Check sheet for the modelled part. Datum: model origin and axes. Units: mm. Face numbers are marked on the shaded views. A direction names the side the tool comes from. Coordinates: 2 decimals unless noted, no trailing zeros. Loops run counter-clockwise (first coordinate to the right, second up) from the corner with the lowest first, then second, coordinate; pieces in that order, holes last. Notation, with made-up numbers: (47.25, -8) -> (89.25, -8) arc R17 ccw to (89.25, 12) -> close; hole circle Ø1 at (31.25, -23). An arc over 180 degrees is marked (long way). Use CSV: the item, a comma, the result in double quotes.
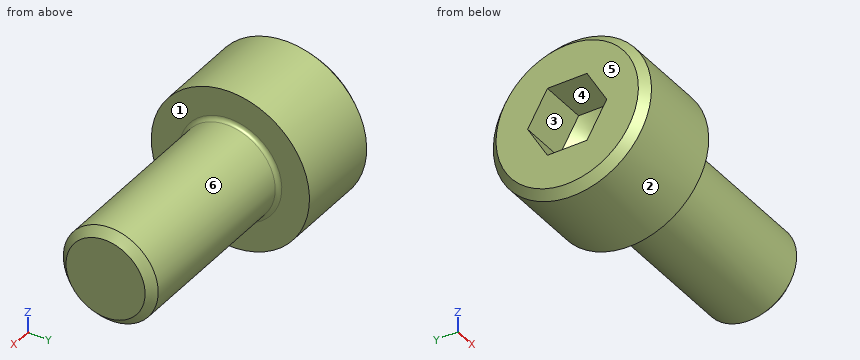
```python
from build123d import *

# Parameters (mm, degrees)
CHAMFER1_SIZE      = 0.5
CUT_EXTRUDE1_DEPTH = 3


with BuildPart() as part:
    # Sketch1 → Revolve1 (revolve)
    with BuildSketch(Plane.XY, mode=Mode.PRIVATE) as revolve1_sk:
        with BuildLine():
            Line((0, 0), (0, 5))
            Line((0, 5), (6, 5))
            Line((6, 5), (6, 3.25))
            ThreePointArc((6, 3.25), (6.073223305, 3.073223305), (6.25, 3))
            Line((6.25, 3), (18, 3))
            Line((18, 3), (18, 0))
            Line((18, 0), (0, 0))
        make_face()
    revolve(revolve1_sk.sketch.rotate(Axis((0, 0, 0), (1, 0, 0)), 90), axis=Axis((0, 0, 0), (1, 0, 0)))

    # Chamfer1
    chamfer1_edges = [part.edges().sort_by_distance(p)[0] for p in [
        (0, 0, -5),
        (18, 0, -3),
    ]]
    chamfer(chamfer1_edges, length=CHAMFER1_SIZE)

    # Sketch2 → Cut-Extrude1 (cut)
    with BuildSketch(Plane.ZY):
        Polygon((0, -2.5), (2.165063509, -1.25), (2.165063509, 1.25), (0, 2.5), (-2.165063509, 1.25), (-2.165063509, -1.25), align=None)
    extrude(amount=-CUT_EXTRUDE1_DEPTH, mode=Mode.SUBTRACT)

    # Sketch3 → Cut-Revolve1 (revolve, cut)
    with BuildSketch(Plane.XY, mode=Mode.PRIVATE) as cut_revolve1_sk:
        Polygon((3, 2.5), (3, 0), (4.5, 0), align=None)
    revolve(cut_revolve1_sk.sketch.rotate(Axis((3, 0, 0), (1, 0, 0)), 270), axis=Axis((3, 0, 0), (1, 0, 0)), mode=Mode.SUBTRACT)


solid = part.part
```
1) Draft check along Z on the marked faces 3, 4, 5 and 6. Enter one of: released by +Z, released by -Z, zero draft, split by the parting line, or undercut.
Answer below:
face 3,"undercut"
face 4,"undercut"
face 5,"zero draft"
face 6,"split by the parting line"
2) Cross-section at A-A on x = 3.75. Record the boundary of the cut face in (y, z).
Answer below:
outline,"circle Ø10 at (0, 0); hole circle Ø2.5 at (0, 0)"
3) Access from +Z, -Z, +X, -X, +Y, -Y to the whole of each face (thin tool, end or side, straight path). Record for the marked faces 1 and 2.
Answer below:
face 1,"+X"
face 2,"+X, -X"
4) Cross-section at B-B on x = 10. Record the boundary of the cut face in (y, z), and give its area (3 significant figures).
Answer below:
outline,"circle Ø6 at (0, 0)"
area,"28.3 mm²"
5) Go/stop test with flat-tipped pins: pin 1 Ø1.5 at (x, y) = (11.5, -3) entering from -Z; pin 2 Ø1.5 at (y, z) = (-3.5, 1) entering from +X; pin 3 Ø3 at (x, y) = (15, -3.5) entering from +Z. Record where each tip stops, or that it passes through.
Answer below:
pin 1,"stops at z = -1.98"
pin 2,"stops at x = 17.61"
pin 3,"stops at z = 2.24"
6) Thickness scan on line 1 along X through (y, z) = (-1.75, -2.75); line 2 along Y through (x, z) = (3.25, 1); line 3 along Y through (x, z) = (2, 0.25). Record the ranges inside material, lowest first. Write a range as from..to.
Answer below:
line 1,"x = 0..6"
line 2,"y = -4.9..-1.83, 1.83..4.9"
line 3,"y = -4.99..-2.36, 2.36..4.99"
